Part model, mm, in its own coordinate system. A direction names the side the tool comes from. Round coordinates to 2 decimals unless told otherwise and drop trailing zeros. Write each loop counter-clockwise with the first axis right and the second up, starting at its lowest first coordinate (ties: lowest second). Pieces come first, ordered by that corner, then holes.
1) Saw through at A-A on z = 35. Write the cut outline in (x, y).
2) Saw through at C-C on y = 78.5. Write the cut outline in (x, z), and give its area (3 significant figures).
3) Saw through at D-D on z = 0. Write the cut outline in (x, y).
4) Pull direction Z, two halves, no side cores. Call faces 1 (the cylindrical face through (1.532, 47.182, 4.864)), 2 (the flat face through (0, 5, 22)), 3 (the cylindrical face through (-7.99, 2.54, 52.15)), 4 (the flat face through (-11, 2, 27)): +Z half, -Z half, draft (parallel to the pull), parting line (faces both ways), or undercut.
5) Which spindle directions (+Z, -Z, +X, -X, +Y, -Y) get a long thin tool onto all of the face, cutting with end or side? Do faces 5 (the flat face through (-9, 10, 34)), 6 (the flat face through (11, 2, 27)), 7 (the cylindrical face through (0.627, 45.455, -14.236)). Say none if no direction does.
6) Flat gauge pins, fed straight in: pin 1 (2.5 mm diameter, centred on y = 2, z = 33.5, fed in from +X); pin 2 (1 mm diameter, centred on x = 5, y = 80.5, fed in from -Z); pin 3 (5.5 mm diameter, centred on y = 3, z = 29, fed in from -X). Where does each tip first touch, or does it go through?
7) Saw through at B-B on x = 0. Write the cut outline in (y, z), and give its area (3 significant figures).
8) Drill centre lines: L1, parallel to X at y = 7.6, z = 35; L2, parallel to Y at x = -1.5, z = -10; L3, parallel to Y at x = -10.5, z = 16.5. Where is each one in solid material? Low to high.
```python
from build123d import *

# Parameters (mm, degrees)
SKETCH1_R           = 14.25
BOSS_EXTRUDE1_DEPTH = 92.2
SKETCH2_R           = 5.1
CUT_EXTRUDE1_DEPTH  = 92.2
SKETCH3_R           = 11.05
CUT_EXTRUDE2_DEPTH  = 4
BOSS_EXTRUDE2_DEPTH = 5
SKETCH6_R           = 8.5
CUT_EXTRUDE3_DEPTH  = 1
FILLET1_R           = 10
BOSS_EXTRUDE3_START = 5
SKETCH7_R           = 10.773488024
SKETCH7_R_2         = 8.5
BOSS_EXTRUDE3_DEPTH = 5


with BuildPart() as part:
    # Sketch1 → Boss-Extrude1 (new body)
    with BuildSketch(Plane(origin=(0, 0, 0), x_dir=(1, 0, 0), z_dir=(0, 1, 0))):
        with Locations(Location((0, 0, 0), (0, 0, 270))):
            Circle(SKETCH1_R)
    extrude(amount=BOSS_EXTRUDE1_DEPTH)

    # Sketch2 → Cut-Extrude1 (cut)
    with BuildSketch(Plane(origin=(0, 92.2, 0), x_dir=(1, 0, 0), z_dir=(0, 1, 0))):
        with Locations(Location((0, 0, 0), (0, 0, 270))):
            Circle(SKETCH2_R)
    extrude(amount=-CUT_EXTRUDE1_DEPTH, mode=Mode.SUBTRACT)

    # Sketch3 → Cut-Extrude2 (cut)
    with BuildSketch(Plane(origin=(0, 92.2, 0), x_dir=(1, 0, 0), z_dir=(0, 1, 0))):
        with Locations(Location((0, 0, 0), (0, 0, 270))):
            Circle(SKETCH3_R)
    extrude(amount=-CUT_EXTRUDE2_DEPTH, mode=Mode.SUBTRACT)

    # Sketch4 → Boss-Extrude2 (add)
    with BuildSketch(Plane.XZ):
        with BuildLine():
            Line((-11, 55), (11, 55))
            Line((11, 55), (11, 9.058835466))
            ThreePointArc((11, 9.058835466), (0, -14.25), (-11, 9.058835466))
            Line((-11, 9.058835466), (-11, 55))
        make_face()
    extrude(amount=-BOSS_EXTRUDE2_DEPTH)

    # Sketch6 → Cut-Extrude3 (cut)
    with BuildSketch(Plane(origin=(0, 5, 0), x_dir=(1, 0, 0), z_dir=(0, 1, 0))):
        with Locations(Location((0, -35, 0), (0, 0, 270))):
            Circle(SKETCH6_R)
    extrude(amount=-CUT_EXTRUDE3_DEPTH, mode=Mode.SUBTRACT)

    # Fillet1
    fillet1_edges = [part.edges().sort_by_distance(p)[0] for p in [
        (-11, 2.5, 55),
        (11, 2.5, 55),
    ]]
    fillet(fillet1_edges, radius=FILLET1_R)

    # Sketch7 → Boss-Extrude3 (add)
    with BuildSketch(Plane(origin=(0, 5, 0), x_dir=(1, 0, 0), z_dir=(0, 1, 0)).offset(BOSS_EXTRUDE3_START)):
        with Locations(Location((0, -35, 0), (0, 0, 90))):
            Circle(SKETCH7_R)
        with Locations(Location((0, -35, 0), (0, 0, 270))):
            Circle(SKETCH7_R_2, mode=Mode.SUBTRACT)
    extrude(amount=-BOSS_EXTRUDE3_DEPTH)


solid = part.part
```
Completed:
1. outline: (-11, 0) - (11, 0) - (11, 5) - (10.77, 5) - (10.77, 10) - (8.5, 10) - (8.5, 4) - (-8.5, 4) - (-8.5, 10) - (-10.77, 10) - (-10.77, 5) - (-11, 5) - close
2. outline: circle Ø28.5 at (0, 0); hole circle Ø10.2 at (0, 0)
2. area: 556 mm2
3. outline: (-14.25, 0) - (14.25, 0) - (14.25, 92.2) - (11.05, 92.2) - (11.05, 88.2) - (5.1, 88.2) - (5.1, 5) - (-5.1, 5) - (-5.1, 88.2) - (-11.05, 88.2) - (-11.05, 92.2) - (-14.25, 92.2) - close
4. face 1: undercut
4. face 2: undercut
4. face 3: +Z half
4. face 4: draft
5. face 5: +Z, +X, -X, +Y
5. face 6: +Z, +X, +Y, -Y
5. face 7: +Y
6. pin 1: stops at x = 11
6. pin 2: stops at z = -13.52
6. pin 3: stops at x = -11
7. outline: (0, -14.25) - (92.2, -14.25) - (92.2, -11.05) - (88.2, -11.05) - (88.2, -5.1) - (5, -5.1) - (5, 5.1) - (88.2, 5.1) - (88.2, 11.05) - (92.2, 11.05) - (92.2, 14.25) - (5, 14.25) - (5, 24.23) - (10, 24.23) - (10, 26.5) - (4, 26.5) - (4, 43.5) - (10, 43.5) - (10, 45.77) - (5, 45.77) - (5, 55) - (0, 55) - close
7. area: 1,900 mm2
8. L1: x = -10.77 to -8.5, 8.5 to 10.77
8. L2: y = 0 to 88.2
8. L3: y = 0 to 5
